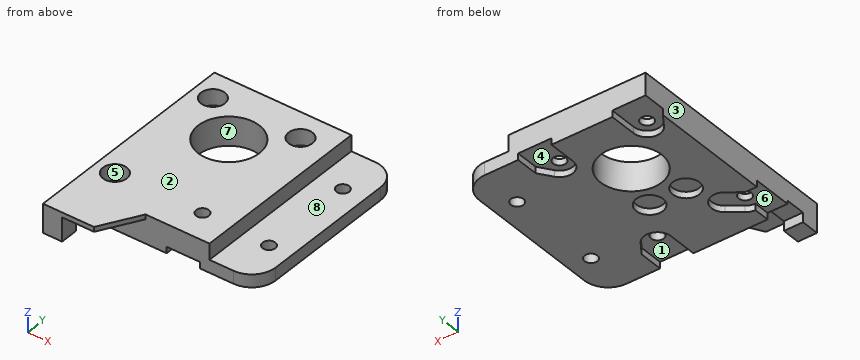
```python
from build123d import *

# Parameters (mm, degrees)
SKETCH1_R           = 9.6
SKETCH1_R_2         = 4.2
BOSS_EXTRUDE1_DEPTH = 2
SKETCH4_W           = 58
SKETCH4_H           = 57.7
SKETCH4_R           = 2
SKETCH4_R_2         = 9.6
BOSS_EXTRUDE3_DEPTH = 2
SKETCH5_R           = 2
CUT_EXTRUDE1_DEPTH  = 4
SKETCH6_W           = 43
SKETCH6_H           = 57.7
SKETCH6_R           = 3.75
SKETCH6_R_2         = 9.6
SKETCH6_R_3         = 2
BOSS_EXTRUDE4_DEPTH = 5
CUT_EXTRUDE2_DEPTH  = 48.972101267
BOSS_EXTRUDE5_DEPTH = 6
BOSS_EXTRUDE6_DEPTH = 1.5


with BuildPart() as part:
    # Sketch1 → Boss-Extrude1 (new body)
    with BuildSketch(Plane.XY):
        with BuildLine():
            Line((38, 28.85), (20, 28.85))
            Line((20, 28.85), (20, 21.79369023))
            Line((20, 21.79369023), (17.201699017, 17.757141063))
            ThreePointArc((17.201699017, 17.757141063), (12.496432266, 16.141438171), (9.55, 20.15))
            Line((9.55, 20.15), (9.55, 28.85))
            Line((9.55, 28.85), (-9.55, 28.85))
            Line((-9.55, 28.85), (-9.55, 20.15))
            ThreePointArc((-9.55, 20.15), (-12.496432266, 16.141438171), (-17.201699017, 17.757141063))
            Line((-17.201699017, 17.757141063), (-20, 21.79369023))
            Line((-20, 21.79369023), (-20, -16.371914064))
            Line((-20, -16.371914064), (-16.312, -16.371914064))
            Line((-16.312, -16.371914064), (-12.349992933, -13.321914064))
            ThreePointArc((-12.349992933, -13.321914064), (-6.459906996, -14.088), (-7.225992933, -19.978085936))
            Line((-7.225992933, -19.978085936), (-11.188, -23.028085936))
            ThreePointArc((-11.188, -23.028085936), (-12.396848296, -23.676050863), (-13.75, -23.9))
            Line((-13.75, -23.9), (-13.75, -28.85))
            Line((-13.75, -28.85), (9.55, -28.85))
            Line((9.55, -28.85), (9.55, -19.7))
            ThreePointArc((9.55, -19.7), (12.496432266, -15.691438171), (17.201699017, -17.307141063))
            Line((17.201699017, -17.307141063), (20, -21.34369023))
            Line((20, -21.34369023), (20, -28.85))
            Line((20, -28.85), (38, -28.85))
            Line((38, -28.85), (38, 28.85))
        make_face()
        with Locations((0, 8.8)):
            Circle(SKETCH1_R, mode=Mode.SUBTRACT)
        with Locations((-5.725, -6.1)):
            Circle(SKETCH1_R_2, mode=Mode.SUBTRACT)
        with Locations((5.725, -6.1)):
            Circle(SKETCH1_R_2, mode=Mode.SUBTRACT)
    extrude(amount=BOSS_EXTRUDE1_DEPTH)

    # Sketch4 → Boss-Extrude3 (add)
    with BuildSketch(Plane.XY.offset(2)):
        with Locations((9, 0)):
            Rectangle(SKETCH4_W, SKETCH4_H)
        with Locations((13.75, -19.7)):
            Circle(SKETCH4_R, mode=Mode.SUBTRACT)
        with Locations((-13.75, 20.15)):
            Circle(SKETCH4_R, mode=Mode.SUBTRACT)
        with Locations((13.75, 20.15)):
            Circle(SKETCH4_R, mode=Mode.SUBTRACT)
        with Locations((-13.75, -19.7)):
            Circle(SKETCH4_R, mode=Mode.SUBTRACT)
        with Locations((0, 8.8)):
            Circle(SKETCH4_R_2, mode=Mode.SUBTRACT)
    extrude(amount=BOSS_EXTRUDE3_DEPTH)

    # Sketch5 → Cut-Extrude1 (cut)
    with BuildSketch(Plane.XY.offset(4)):
        with Locations((31, 15)):
            Circle(SKETCH5_R)
        with Locations((31, -15)):
            Circle(SKETCH5_R)
    extrude(amount=-CUT_EXTRUDE1_DEPTH, mode=Mode.SUBTRACT)

    # Sketch6 → Boss-Extrude4 (add)
    with BuildSketch(Plane.XY.offset(4)):
        with Locations((1.5, 0)):
            Rectangle(SKETCH6_W, SKETCH6_H)
        with Locations((-13.75, -19.7)):
            Circle(SKETCH6_R, mode=Mode.SUBTRACT)
        with Locations((0, 8.8)):
            Circle(SKETCH6_R_2, mode=Mode.SUBTRACT)
        with Locations((-13.75, 20.15)):
            Circle(SKETCH6_R, mode=Mode.SUBTRACT)
        with Locations((13.75, 20.15)):
            Circle(SKETCH6_R, mode=Mode.SUBTRACT)
        with Locations((13.75, -19.7)):
            Circle(SKETCH6_R_3, mode=Mode.SUBTRACT)
    extrude(amount=BOSS_EXTRUDE4_DEPTH)

    # Sketch7 → Cut-Extrude2 (cut, through all)
    with BuildSketch(Plane.XY.offset(4)):
        with BuildLine():
            Line((30.5, 28.85), (38, 28.85))
            Line((38, 28.85), (38, 21.35))
            ThreePointArc((38, 21.35), (35.803300859, 26.653300859), (30.5, 28.85))
        make_face()
        with BuildLine():
            Line((38, -28.85), (38, -21.35))
            ThreePointArc((38, -21.35), (35.803300859, -26.653300859), (30.5, -28.85))
            Line((30.5, -28.85), (38, -28.85))
        make_face()
    extrude(amount=-CUT_EXTRUDE2_DEPTH, mode=Mode.SUBTRACT)

    # Sketch9 → Boss-Extrude5 (add)
    with BuildSketch(Plane.ZY.offset(20)):
        Polygon((9, -28.85), (9, -40.85), (0, -40.85), (0, -35.15), (3, -35.15), (3, -28.85), align=None)
    extrude(amount=-BOSS_EXTRUDE5_DEPTH)

    # Sketch10 → Boss-Extrude6 (add)
    with BuildSketch(Plane.XY.offset(9)):
        Polygon((-14, -40.85), (-4, -40.85), (2.92820323, -28.85), (-14, -28.85), align=None)
    extrude(amount=-BOSS_EXTRUDE6_DEPTH)


solid = part.part
```
Read the model definition and answer for the solid it produces. Units are mm, in the model's axes. Face numbers are marked on the shaded views. A direction names the side the tool comes from. Coordinates: 2 decimals unless noted, no trailing zeros. Loops run counter-clockwise (first coordinate to the right, second up) from the corner with the lowest first, then second, coordinate; pieces in that order, holes last. Notation, with made-up numbers: (50, 74) -> (87, 74) arc R11 cw to (87, 82) -> close; hole circle Ø4 at (-8.5, 35). An arc over 180 degrees is marked (long way). Return JSON: item names as keys, results as strings.
Item 1: Find section B-B (x = 13.75). Determine the outline of the cut face in (y, z).
Answers:
{"outline": "(-28.85, 2) -> (-21.7, 2) -> (-21.7, 9) -> (-28.85, 9) -> close; (-17.7, 2) -> (-15.5, 2) -> (-15.5, 0) -> (15.95, 0) -> (15.95, 2) -> (18.15, 2) -> (18.15, 4) -> (16.4, 4) -> (16.4, 9) -> (-17.7, 9) -> close; (22.15, 2) -> (28.85, 2) -> (28.85, 9) -> (23.9, 9) -> (23.9, 4) -> (22.15, 4) -> close"}
Item 2: Find section D-D (y = -6.1). Determine the outline of the cut face in (x, z) (3 decimals), plus the area to 3 significant figures.
Answers:
{"outline": "(-20, 0) -> (-9.925, 0) -> (-9.925, 2) -> (-1.525, 2) -> (-1.525, 0) -> (1.525, 0) -> (1.525, 2) -> (9.925, 2) -> (9.925, 0) -> (38, 0) -> (38, 4) -> (23, 4) -> (23, 9) -> (-20, 9) -> close", "area": "413 mm2"}
Item 3: Find the intervals of material crossed by probe 1 along Y at (x, z) = (-13.75, 5.2); probe 2 along Y at (x, z) = (-13.75, 3.45); probe 3 along Y at (x, z) = (0, 6.75), in increasing order.
Answers:
{"probe 1": "y = -28.85 to -23.45, -15.95 to 16.4, 23.9 to 28.85", "probe 2": "y = -28.85 to -21.7, -17.7 to 18.15, 22.15 to 28.85", "probe 3": "y = -28.85 to -0.8, 18.4 to 28.85"}
Item 4: For a pull along X with two mould halves and no side action, classify the marked faces 1, 2 and 3 as +X half, -X half, draft (parallel to the pull), parting line (faces both ways), or undercut.
Answers:
{"face 1": "undercut", "face 2": "draft", "face 3": "-X half"}
Item 5: For the marked faces 4, 5, 6, 7 and 8, determine the directions among +Z, -Z, +X, -X, +Y, -Y from which every point of the face is accessible in a straight line to the end or side of a thin tool.
Answers:
{"face 4": "-Z, +Y", "face 5": "+Z", "face 6": "-Z", "face 7": "+Z, -Z", "face 8": "+Z, +X, +Y, -Y"}
Item 6: Find section A-A (z = 5). Determine the outline of the cut face in (x, y), plus the area to 3 significant figures.
Answers:
{"outline": "(-20, -40.85) -> (-14, -40.85) -> (-14, -28.85) -> (23, -28.85) -> (23, 28.85) -> (-20, 28.85) -> close; hole circle Ø7.5 at (-13.75, -19.7); hole circle Ø7.5 at (-13.75, 20.15); hole circle Ø19.2 at (0, 8.8); hole circle Ø7.5 at (13.75, 20.15); hole circle Ø4 at (13.75, -19.7)", "area": "2,120 mm2"}
Item 7: Find section C-C (y = 7). Determine the outline of the cut face in (x, z).
Answers:
{"outline": "(-20, 0) -> (-9.43, 0) -> (-9.43, 9) -> (-20, 9) -> close; (9.43, 0) -> (38, 0) -> (38, 4) -> (23, 4) -> (23, 9) -> (9.43, 9) -> close"}
Item 8: Flat-ended cylindrical pins translate along their axes: P1, Ø1.6, axis at y = -27, z = 1, coming from the -X side; P2, Ø5, axis at x = 31, y = -15, coming from the +Z side; P3, Ø2.5, axis at x = -17.5, z = 1.5, coming from the +Y side; P4, Ø6.5, axis at x = -17.5, y = -31.5, coming from the -Z side. Find the tip coordinate at first contact, or state that the pin passes through.
Answers:
{"P1": "stops at x = -13.75", "P2": "stops at z = 4", "P3": "stops at y = 28.85", "P4": "stops at z = 2"}
